The model under review builds one solid part; all positions refer to its coordinate system, in mm. A direction names the side the tool comes from. Round coordinates to 2 decimals unless told otherwise and drop trailing zeros. Order: outer loops, then holes, each group sorted by start corner. A loop starts at its lowest first (then second) coordinate and runs counter-clockwise, first axis right, second up. Notation, with made-up numbers: (-26, -6.5) -> (-17, -6.5) arc R15 ccw to (-17, -1.5) -> close; hole circle Ø11 at (48, 19). An arc over 180 degrees is marked (long way). Use a Markdown table: item, result. Add a question column.
Autodesk Inventor part; units mm, degrees
ref_plane "YZ Plane" through (0, 0, 0) normal (1, 0, 0) x (0, 1, 0)
ref_plane "XZ Plane" through (0, 0, 0) normal (0, 1, 0) x (-1, 0, 0)
ref_plane "XY Plane" through (0, 0, 0) normal (0, 0, 1) x (1, 0, 0)
sketch "Sketch1" plane through (0, 0, 0) normal (0, 0, 1) x (1, 0, 0)
  circle A0 centre (0, 0) radius 19
  dimension "d1" = 38
extrude "Extrusion1" add sketch "Sketch1" along normal blind 50
sketch "Sketch2" plane through (0, 0, 50) normal (0, 0, 1) x (1, 0, 0)
  circle A0 centre (0, 12) radius 1.25
  circle A1 centre (0, -12) radius 1.25
  point P0 (0, 0)
  dimension "d4" = 12
  dimension "d5" = 12
  dimension "d6" = 2.5
  dimension "d7" = 2.5
extrude "Extrusion2" add sketch "Sketch2" along normal blind 2 contours A0
sketch "Sketch3" plane through (0, 0, 50) normal (0, 0, 1) x (1, 0, 0)
  circle A0 centre (0, -12) radius 1.25
  point P0 (0, 0)
  dimension "d10" = 12
  dimension "d11" = 2.5
extrude "Extrusion3" add sketch "Sketch3" along normal blind 2
properties part number "motor"
Q1. Add section D-D, the plane y = 0. Give the boundary of the cut face in (x, z), then the cut area to 3 significant figures.
Q2. Add section A-A, the plane x = 0. Give the boundary of the cut face in (y, z), then the cut area to 3 significant figures.
Q3. For faces 1 (the face through (-0.16, 10.76, 50.99)), 2 (the face through (8.767, 16.856, 24.65)), list the 3-axis set-ups (+Z, -Z, +X, -X, +Y, -Y) from which the entire face can be reached by the end or side of a thin tool; tool diameter is ignored.
Q4. Add section B-B, the plane y = 12. Give the boundary of the cut face in (x, z).
Q5. For pin 1 (4 mm diameter, centred on y = -8.5, z = 46.5, fed in from +X); pin 2 (10 mm diameter, centred on x = -13.5, z = 13.5, fed in from -Y); pin 3 (3 mm diameter, centred on y = 12, z = 21, fed in from -X), all flat-tipped, find the tip position at first contact; note any pin that passes through.
Q6. To check wall thickness, follow line 1 along Z through (x, y) = (-3.5, -7); line 2 along Y through (x, z) = (0, 2.5); line 3 along X through (y, z) = (4, 13). State the ranges of each line that lie inside material, in increasing order.
Q7. Add section C-C, the plane z = 32. Give the boundary of the cut face in (x, y).
Return value:
| question | item | result |
|---|---|---|
| 1 | outline | (-19, 0) -> (19, 0) -> (19, 50) -> (-19, 50) -> close |
| 1 | area | 1,900 mm² |
| 2 | outline | (-19, 0) -> (19, 0) -> (19, 50) -> (13.25, 50) -> (13.25, 52) -> (10.75, 52) -> (10.75, 50) -> (-10.75, 50) -> (-10.75, 52) -> (-13.25, 52) -> (-13.25, 50) -> (-19, 50) -> close |
| 2 | area | 1,910 mm² |
| 3 | face 1 | +Z |
| 3 | face 2 | +Z, -Z |
| 4 | outline | (-14.73, 0) -> (14.73, 0) -> (14.73, 50) -> (1.25, 50) -> (1.25, 52) -> (-1.25, 52) -> (-1.25, 50) -> (-14.73, 50) -> close |
| 5 | pin 1 | x = 17.85 |
| 5 | pin 2 | y = -16.99 |
| 5 | pin 3 | x = -15.84 |
| 6 | line 1 | 0 to 50 |
| 6 | line 2 | -19 to 19 |
| 6 | line 3 | -18.57 to 18.57 |
| 7 | outline | circle Ø38 at (0, 0) |
